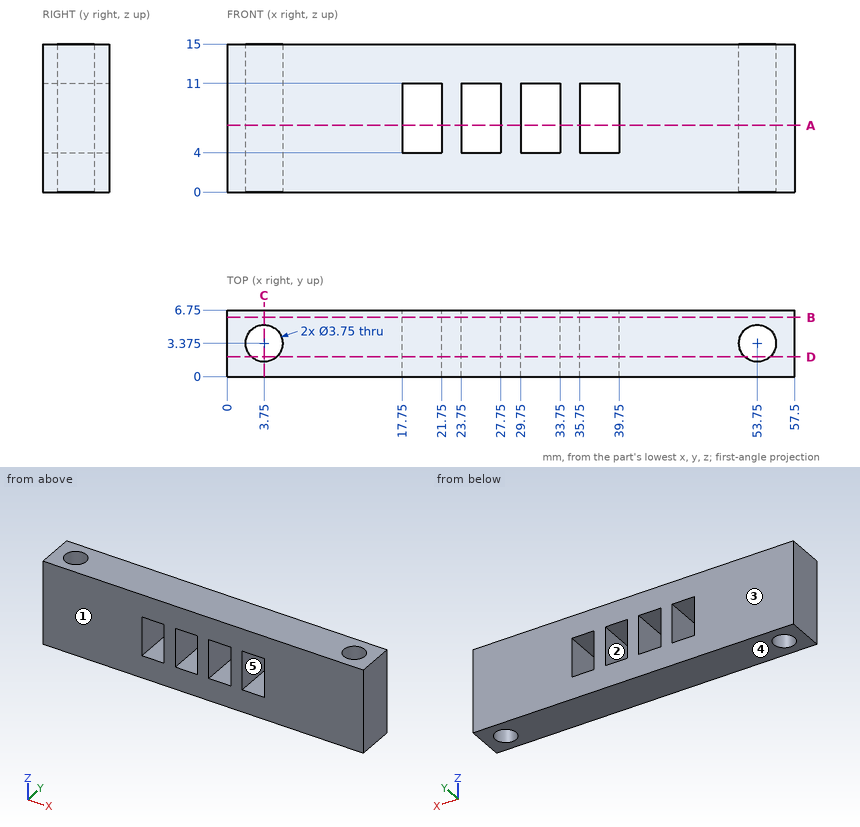
Design review of the part shown in the three views and the two pictorial views. Dimensions are in mm from the part's minimum x, y and z. A direction names the side the tool comes from. Round coordinates to 2 decimals unless told otherwise and drop trailing zeros. Order: outer loops, then holes, each group sorted by start corner. A loop starts at its lowest first (then second) coordinate and runs counter-clockwise, first axis right, second up. Notation, with made-up numbers: (-3, 27) - (54, 27) arc R15 ccw to (54, 54) - close; hole circle Ø1 at (11.25, 48). An arc over 180 degrees is marked (long way). Answer in a Markdown table with one row per item.
(1) Machinability: for the marked faces 1 and 2, which of the approach directions +Z, -Z, +X, -X, +Y, -Y give a long, thin tool a straight path to every point of the face, cutting with its end or side? Answer none if there is none.
Result set:
| item | result |
|---|---|
| face 1 | +Z, -Z, +X, -X, -Y |
| face 2 | +Y, -Y |
(2) For line 1 (X direction, y = 6.25, z = 10.5); line 2 (X direction, y = 3.5, z = 2.75); line 3 (Z direction, x = 19, y = 1.5), list the stretches that pass through material, from the lowest coordinate up. Write a range as from..to.
Result set:
| item | result |
|---|---|
| line 1 | x = 0..17.75, 21.75..23.75, 27.75..29.75, 33.75..35.75, 39.75..57.5 |
| line 2 | x = 0..1.88, 5.62..51.88, 55.62..57.5 |
| line 3 | z = 0..4, 11..15 |
(3) Take a section at C-C on x = 3.75. Write out the cut boundary in (y, z).
Result set:
| item | result |
|---|---|
| outline | (0, 0) - (1.5, 0) - (1.5, 15) - (0, 15) - close; (5.25, 0) - (6.75, 0) - (6.75, 15) - (5.25, 15) - close |
(4) Take a section at D-D on y = 2. Write out the cut boundary in (x, z), plus the area to 3 significant figures.
Result set:
| item | result |
|---|---|
| outline | (0, 0) - (2.48, 0) - (2.48, 15) - (0, 15) - close; (5.02, 0) - (52.48, 0) - (52.48, 15) - (5.02, 15) - close; (55.02, 0) - (57.5, 0) - (57.5, 15) - (55.02, 15) - close; hole (17.75, 4) - (21.75, 4) - (21.75, 11) - (17.75, 11) - close; hole (23.75, 4) - (27.75, 4) - (27.75, 11) - (23.75, 11) - close; hole (29.75, 4) - (33.75, 4) - (33.75, 11) - (29.75, 11) - close; hole (35.75, 4) - (39.75, 4) - (39.75, 11) - (35.75, 11) - close |
| area | 674 mm2 |
(5) Mouldability with a two-part tool opening along Z and no side actions: class the marked faces 3, 4 and 5 as released by +Z, released by -Z, zero draft, split by the parting line, or undercut.
Result set:
| item | result |
|---|---|
| face 3 | zero draft |
| face 4 | released by -Z |
| face 5 | undercut |
(6) Take a section at A-A on z = 6.75. Write out the cut boundary in (x, y) (3 decimals), plus the area to 3 significant figures.
Result set:
| item | result |
|---|---|
| outline | (0, 0) - (17.75, 0) - (17.75, 6.75) - (0, 6.75) - close; (21.75, 0) - (23.75, 0) - (23.75, 6.75) - (21.75, 6.75) - close; (27.75, 0) - (29.75, 0) - (29.75, 6.75) - (27.75, 6.75) - close; (33.75, 0) - (35.75, 0) - (35.75, 6.75) - (33.75, 6.75) - close; (39.75, 0) - (57.5, 0) - (57.5, 6.75) - (39.75, 6.75) - close; hole circle Ø3.75 at (3.75, 3.375); hole circle Ø3.75 at (53.75, 3.375) |
| area | 258 mm2 |
(7) Take a section at B-B on y = 6. Write out the cut boundary in (x, z).
Result set:
| item | result |
|---|---|
| outline | (0, 0) - (57.5, 0) - (57.5, 15) - (0, 15) - close; hole (17.75, 4) - (21.75, 4) - (21.75, 11) - (17.75, 11) - close; hole (23.75, 4) - (27.75, 4) - (27.75, 11) - (23.75, 11) - close; hole (29.75, 4) - (33.75, 4) - (33.75, 11) - (29.75, 11) - close; hole (35.75, 4) - (39.75, 4) - (39.75, 11) - (35.75, 11) - close |
